Autodesk Inventor part; units mm, degrees
ref_plane "Work Plane6" through (0, -199.5457, 0) normal (0, -0.0454077, 0.9989685) x (1, 0, 0)
ref_plane "Work Plane7" through (0, 0, 0) normal (0, 0, 1) x (1, 0, 0)
ref_plane "Work Plane9" through (125, -1279.7641, -134.7549) normal (0, -1, 0) x (-1, 0, 0)
ref_plane "Work Plane6" through (0, -199.5457, 0) normal (0, -0.0454077, 0.9989685) x (1, 0, 0)
sketch "Sketch4" plane through (0, -199.5457, 0) normal (0, -0.0454077, 0.9989685) x (1, 0, 0)
  line L0 (220, 0) -> (220, -976.9106)
  line L1 (0, 0) -> (220, 0)
  line L2 (0, 0) -> (0, -976.9106)
  line L3 (0, -976.9106) -> (220, -976.9106)
  point P0 (0, 199.3399)
extrude "Plate4" add sketch "Sketch4" against normal blind 1.5
ref_plane "Work Plane7" through (0, 0, 0) normal (0, 0, 1) x (1, 0, 0)
sketch "Sketch5" plane through (0, 0, 0) normal (0, 0, -1) x (1, 0, 0)
  line L0 (0, -166.5116) -> (220, -166.5116)
  line L1 (220, -166.5116) -> (220, 0.4543)
  line L2 (220, 0.4543) -> (0, 0.4543)
  line L3 (0, 0.4543) -> (0, -166.5116)
edge flange "Flange3" height 200 angle 90 thickness 1.5 bend radius 1.5 thickness toward (0, 0, -1) relief tear relief width 1.5 relief depth 0.75 edges at (110, -199.4776, -1.4985) wall of the first edge with corners at (0, -166.5116, 0) (220, -166.5116, 0) (220, 0.4543, 0) (0, 0.4543, 0)
bend "Bend3"
corner "Corner3"
sketch "Sketch6" plane through (0, 0.4543, 0) normal (0, 0, 1) x (1, 0, 0)
  arc A0 (220, -130.306) -> (201.1417, -102.4517) centre (190, -130.306) ccw
  line L0 (0, -21.995) -> (201.1417, -102.4517)
  line L1 (0, -21.995) -> (0, -200)
  line L2 (0, -200) -> (220, -200)
  line L3 (220, -130.306) -> (220, -200)
  line L4 (0, -199.9319) -> (220, -199.9319)
  line L5 (220, 0) -> (220, -199.9319)
  line L6 (0, 0) -> (220, 0)
  line L7 (0, -199.9319) -> (0, 0)
  point P0 (0, -0.4543)
  point P1 (220, -130.306)
extrude "Extrusion1" cut sketch "Sketch6" against normal through all contours A0 L0 L7 L6 L5
ref_plane "Work Plane9" through (125, -1279.7641, -134.7549) normal (0, -1, 0) x (-1, 0, 0)
sketch "Sketch8" plane through (125, -1279.7641, -134.7549) normal (0, 1, 0) x (-1, 0, 0)
  line L0 (-95, -84.1525) -> (125, -84.1525)
  line L1 (125, -84.1525) -> (125, 29.3459)
  line L2 (125, 29.3459) -> (-95, 29.3459)
  line L3 (-95, 29.3459) -> (-95, -84.1525)
edge flange "Flange5" height 115 angle 90 thickness 1.5 bend radius 108.5 thickness toward (0, 1, 0) relief tear relief width 1.5 relief depth 0.75 edges at (110, -1175.3806, -45.8577) wall of the first edge with corners at (220, -1279.7641, -50.6024) (0, -1279.7641, -50.6024) (0, -1279.7641, -164.1008) (220, -1279.7641, -164.1008)
bend "Bend5"
corner "Corner5"
ref_plane "Work Plane8" through (125, -1278.2641, -134.7549) normal (0, -1, 0) x (-1, 0, 0)
sketch "Sketch9" plane through (220, -1279.7641, -164.1008) normal (1, 0, 0) x (0, 0, -1)
  line L0 (-9.8864, 1.5) -> (-9.8864, 0)
  arc A0 (-118.2745, 105.0733) -> (-9.8864, 1.5) centre (-9.8864, 110) ccw
  line L1 (-119.773, 105.0052) -> (-118.2745, 105.0733)
  arc A1 (-119.773, 105.0052) -> (-9.8864, 0) centre (-9.8864, 110) ccw
  line L2 (-9.8864, 1.5) -> (-9.8864, 0)
  line L3 (-9.8864, 0) -> (0, 0)
  line L4 (0, 1.5) -> (0, 0)
  line L5 (-9.8864, 1.5) -> (0, 1.5)
  line L6 (-29.3211, 1.7305) -> (-29.0561, 3.2069)
  point P0 (-164.1008, 1279.7641)
sketch3d "3D Sketch1"
sketch "Sketch1" plane through (0, 0, 0) normal (0, 0, 1) x (1, 0, 0)
  line L0 (1250.1265, -201.1417) -> (1330.5832, 0)
  line L1 (0, 0) -> (1330.5832, 0)
  line L2 (0, -220) -> (0, 0)
  line L3 (1222.2722, -220) -> (0, -220)
  arc A0 (1222.2722, -220) -> (1250.1265, -201.1417) centre (1222.2722, -190) ccw
equation "\"d22\" = Thickness"
equation "\"d23\" = BendReliefWidth"
equation "\"d24\" = BendReliefDepth"
equation "\"d25\" = MinimumRemnant"
equation "\"d26\" = TransitionRadius"
equation "\"d29\" = BendRadius"
equation "\"d30\" = CornerReliefSize"
equation "\"d31\" = GapSize"
equation "\"d32\" = JacobiRadiusSize"
equation "\"d46\" = BendReliefWidth"
equation "\"d47\" = BendReliefDepth"
equation "\"d48\" = MinimumRemnant"
equation "\"d49\" = TransitionRadius"
equation "\"d53\" = CornerReliefSize"
equation "\"d54\" = GapSize"
equation "\"d55\" = JacobiRadiusSize"
equation "\"BendRadius\" = Thickness"
equation "\"BendReliefWidth\" = Thickness"
equation "\"BendReliefDepth\" = 0.5 * Thickness"
equation "\"CornerReliefSize\" = 4 * Thickness"
equation "\"MinimumRemnant\" = 2 * Thickness"
equation "\"TransitionRadius\" = BendRadius"
equation "\"JacobiRadiusSize\" = BendRadius"
equation "\"GapSize\" = Thickness"
properties part number "CARCASA_ALUM_3"
Geometry: final body of the model. Coordinates: model frame, mm. Coordinates: 2 decimals unless noted, no trailing zeros. Loops run counter-clockwise (first coordinate to the right, second up) from the corner with the lowest first, then second, coordinate; pieces in that order, holes last. Notation, with made-up numbers: M 20,-26.5 L 42,-26.5 A31 cw 42,9.5 Z; hole C 41,76 d1. An arc over 180 degrees is marked long. Put each result on its own line as item: value.
(1) Cut plane D-D on x = 56.5. Return the cut outline in (y, z), then the cut area to 3 significant figures.
Answer sheet:
outline: M -1279.76,-164.1 L -1278.26,-164.1 L -1278.26,-154.21 A108.5 cw -1174.69,-45.83 L -199.55,-1.5 A1.5 cw -199.48,-1.5 L -44.14,-1.5 L -44.14,0 L -199.48,0 A3 ccw -199.61,0 L -1174.76,-44.33 A110 ccw -1279.76,-154.21 Z
area: 1,960 mm^2
(2) Cut plane C-C on z = -71. Return the cut outline in (x, y).
Answer sheet:
outline: M 0,-1241.7 L 220,-1241.7 L 220,-1239.39 L 0,-1239.39 Z
(3) First-contact query: pin 1 (4 mm diameter, centred on x = 184.5, z = -142, fed in from +Y); pin 2 (12 mm diameter, centred on x = 138.5, z = -143, fed in from -Y); pin 3 (2 mm diameter, centred on x = 91.5, y = -289, fed in from -Z). Flat tips, straight axial feed; report the tip coordinate or a pass-through.
Answer sheet:
pin 1: stops at y = -1277.33
pin 2: stops at y = -1279.64
pin 3: stops at z = -5.61
(4) Cut plane A-A on x = 127. Return the cut outline in (y, z), then the cut area to 3 significant figures.
Answer sheet:
outline: M -1279.76,-164.1 L -1278.26,-164.1 L -1278.26,-154.21 A108.5 cw -1174.69,-45.83 L -199.55,-1.5 A1.5 cw -199.48,-1.5 L -72.34,-1.5 L -72.34,0 L -199.48,0 A3 ccw -199.61,0 L -1174.76,-44.33 A110 ccw -1279.76,-154.21 Z
area: 1,920 mm^2
(5) Draft query along Z for faces 1 (the face through (99.163, -61.206, -0.74)), 2 (the face through (112, -132, -1.5)), 3 (the face through (108.46, -680.36, -21.855)). Return one class per face: pulls with the +Z half, pulls with the -Z half, needs draft (parallel to the pull), parting line crosses it, or undercut.
Answer sheet:
face 1: needs draft
face 2: pulls with the -Z half
face 3: pulls with the +Z half
(6) Material intervals for probe 1 along Y at (x, z) = (188, -73); probe 2 along Z at (x, y) = (159, -190); probe 3 along Z at (x, y) = (132, -903), sorted ascending.
Answer sheet:
probe 1: y = -1243.95 to -1241.71
probe 2: z = -1.5 to 0
probe 3: z = -33.48 to -31.98
(7) Cut plane B-B on y = -155. Return the cut outline in (x, z), then the cut area to 3 significant figures.
Answer sheet:
outline: M 0,-1.5 L 220,-1.5 L 220,0 L 0,0 Z
area: 330 mm^2
